from build123d import *

# Parameters (mm, degrees)
F0_R     = 43
F0_R_2   = 40
F0_R_3   = 4.25
F1_DEPTH = 2
F2_DEPTH = 160
F4_DEPTH = 155


with BuildPart() as f1:
    # F0 (on Top) → F1 (new body)
    with BuildSketch(Plane.XY):
        Circle(F0_R)
        Circle(F0_R_2, mode=Mode.SUBTRACT)
        Circle(F0_R_2)
        Circle(F0_R_3, mode=Mode.SUBTRACT)
    extrude(amount=F1_DEPTH)

    # F0 (on Top) → F2 (join)
    with BuildSketch(Plane.XY):
        Circle(F0_R)
        Circle(F0_R_2, mode=Mode.SUBTRACT)
    extrude(amount=F2_DEPTH)

    # F3 (on face) → F4 (cut)
    with BuildSketch(Plane.XY.offset(160)):
        with BuildLine():
            ThreePointArc((-17.935173408, 35.7537348374), (-15.3073372946, 36.9551813005), (-12.5996256178, 37.9637910948))
            Line((-12.5996256178, 37.9637910948), (-15.1896329803, 38.9425798282))
            Line((-15.1896329803, 38.9425798282), (-16.7958697893, 38.2772547575))
            Line((-16.7958697893, 38.2772547575), (-17.935173408, 35.7537348374))
        make_face()
        with BuildLine():
            ThreePointArc((-10.6153464373, 38.5657156036), (-7.8036128806, 39.2314112161), (-4.9511591149, 39.6923925132))
            Line((-4.9511591149, 39.6923925132), (-7.300448003, 41.1576594658))
            Line((-7.300448003, 41.1576594658), (-9.0056199043, 40.8184796861))
            Line((-9.0056199043, 40.8184796861), (-10.6153464373, 38.5657156036))
        make_face()
        with BuildLine():
            Line((-0.8692890969, 41.7910733317), (-2.8875776562, 39.895637547))
            ThreePointArc((-2.8875776562, 39.895637547), (0, 40), (2.8875776562, 39.895637547))
            Line((2.8875776562, 39.895637547), (0.8692890969, 41.7910733317))
            Line((0.8692890969, 41.7910733317), (-0.8692890969, 41.7910733317))
        make_face()
        with BuildLine():
            Line((7.300448003, 41.1576594658), (4.9511591149, 39.6923925132))
            ThreePointArc((4.9511591149, 39.6923925132), (7.8036128806, 39.2314112161), (10.6153464373, 38.5657156036))
            Line((10.6153464373, 38.5657156036), (9.0056199043, 40.8184796861))
            Line((9.0056199043, 40.8184796861), (7.300448003, 41.1576594658))
        make_face()
        with BuildLine():
            Line((15.1896329803, 38.9425798282), (12.5996256178, 37.9637910948))
            ThreePointArc((12.5996256178, 37.9637910948), (15.3073372946, 36.9551813005), (17.935173408, 35.7537348374))
            Line((17.935173408, 35.7537348374), (16.7958697893, 38.2772547575))
            Line((16.7958697893, 38.2772547575), (15.1896329803, 38.9425798282))
        make_face()
        with BuildLine():
            ThreePointArc((-24.5657617227, 31.5677580924), (-22.2228093208, 33.2587844921), (-19.7638955741, 34.7762624751))
            Line((-19.7638955741, 34.7762624751), (-22.4950888807, 35.2309586869))
            Line((-22.4950888807, 35.2309586869), (-23.9406638174, 34.2650563947))
            Line((-23.9406638174, 34.2650563947), (-24.5657617227, 31.5677580924))
        make_face()
        with BuildLine():
            ThreePointArc((-30.2523015911, 26.1686501073), (-28.2842712475, 28.2842712475), (-26.1686501073, 30.2523015911))
            Line((-26.1686501073, 30.2523015911), (-28.9360711307, 30.1654315611))
            Line((-28.9360711307, 30.1654315611), (-30.1654315611, 28.9360711307))
            Line((-30.1654315611, 28.9360711307), (-30.2523015911, 26.1686501073))
        make_face()
        with BuildLine():
            ThreePointArc((-34.7762624751, 19.7638955741), (-33.2587844921, 22.2228093208), (-31.5677580924, 24.5657617227))
            Line((-31.5677580924, 24.5657617227), (-34.2650563947, 23.9406638174))
            Line((-34.2650563947, 23.9406638174), (-35.2309586869, 22.4950888807))
            Line((-35.2309586869, 22.4950888807), (-34.7762624751, 19.7638955741))
        make_face()
        with BuildLine():
            ThreePointArc((-37.9637910948, 12.5996256178), (-36.9551813005, 15.3073372946), (-35.7537348374, 17.935173408))
            Line((-35.7537348374, 17.935173408), (-38.2772547575, 16.7958697893))
            Line((-38.2772547575, 16.7958697893), (-38.9425798282, 15.1896329803))
            Line((-38.9425798282, 15.1896329803), (-37.9637910948, 12.5996256178))
        make_face()
        with BuildLine():
            ThreePointArc((-39.6923925132, 4.9511591149), (-39.2314112161, 7.8036128806), (-38.5657156036, 10.6153464373))
            Line((-38.5657156036, 10.6153464373), (-40.8184796861, 9.0056199043))
            Line((-40.8184796861, 9.0056199043), (-41.1576594658, 7.300448003))
            Line((-41.1576594658, 7.300448003), (-39.6923925132, 4.9511591149))
        make_face()
        with BuildLine():
            Line((22.4950888807, 35.2309586869), (19.7638955741, 34.7762624751))
            ThreePointArc((19.7638955741, 34.7762624751), (22.2228093208, 33.2587844921), (24.5657617227, 31.5677580924))
            Line((24.5657617227, 31.5677580924), (23.9406638174, 34.2650563947))
            Line((23.9406638174, 34.2650563947), (22.4950888807, 35.2309586869))
        make_face()
        with BuildLine():
            Line((28.9360711307, 30.1654315611), (26.1686501073, 30.2523015911))
            ThreePointArc((26.1686501073, 30.2523015911), (28.2842712475, 28.2842712475), (30.2523015911, 26.1686501073))
            Line((30.2523015911, 26.1686501073), (30.1654315611, 28.9360711307))
            Line((30.1654315611, 28.9360711307), (28.9360711307, 30.1654315611))
        make_face()
        with BuildLine():
            Line((34.2650563947, 23.9406638174), (31.5677580924, 24.5657617227))
            ThreePointArc((31.5677580924, 24.5657617227), (33.2587844921, 22.2228093208), (34.7762624751, 19.7638955741))
            Line((34.7762624751, 19.7638955741), (35.2309586869, 22.4950888807))
            Line((35.2309586869, 22.4950888807), (34.2650563947, 23.9406638174))
        make_face()
        with BuildLine():
            Line((38.2772547575, 16.7958697893), (35.7537348374, 17.935173408))
            ThreePointArc((35.7537348374, 17.935173408), (36.9551813005, 15.3073372946), (37.9637910948, 12.5996256178))
            Line((37.9637910948, 12.5996256178), (38.9425798282, 15.1896329803))
            Line((38.9425798282, 15.1896329803), (38.2772547575, 16.7958697893))
        make_face()
        with BuildLine():
            ThreePointArc((-39.895637547, -2.8875776562), (-40, 0), (-39.895637547, 2.8875776562))
            Line((-39.895637547, 2.8875776562), (-41.7910733317, 0.8692890969))
            Line((-41.7910733317, 0.8692890969), (-41.7910733317, -0.8692890969))
            Line((-41.7910733317, -0.8692890969), (-39.895637547, -2.8875776562))
        make_face()
        with BuildLine():
            ThreePointArc((-38.5657156036, -10.6153464373), (-39.2314112161, -7.8036128806), (-39.6923925132, -4.9511591149))
            Line((-39.6923925132, -4.9511591149), (-41.1576594658, -7.300448003))
            Line((-41.1576594658, -7.300448003), (-40.8184796861, -9.0056199043))
            Line((-40.8184796861, -9.0056199043), (-38.5657156036, -10.6153464373))
        make_face()
        with BuildLine():
            ThreePointArc((-35.7537348374, -17.935173408), (-36.9551813005, -15.3073372946), (-37.9637910948, -12.5996256178))
            Line((-37.9637910948, -12.5996256178), (-38.9425798282, -15.1896329803))
            Line((-38.9425798282, -15.1896329803), (-38.2772547575, -16.7958697893))
            Line((-38.2772547575, -16.7958697893), (-35.7537348374, -17.935173408))
        make_face()
        with BuildLine():
            ThreePointArc((-31.5677580924, -24.5657617227), (-33.2587844921, -22.2228093208), (-34.7762624751, -19.7638955741))
            Line((-34.7762624751, -19.7638955741), (-35.2309586869, -22.4950888807))
            Line((-35.2309586869, -22.4950888807), (-34.2650563947, -23.9406638174))
            Line((-34.2650563947, -23.9406638174), (-31.5677580924, -24.5657617227))
        make_face()
        with BuildLine():
            ThreePointArc((-26.1686501073, -30.2523015911), (-28.2842712475, -28.2842712475), (-30.2523015911, -26.1686501073))
            Line((-30.2523015911, -26.1686501073), (-30.1654315611, -28.9360711307))
            Line((-30.1654315611, -28.9360711307), (-28.9360711307, -30.1654315611))
            Line((-28.9360711307, -30.1654315611), (-26.1686501073, -30.2523015911))
        make_face()
        with BuildLine():
            ThreePointArc((-19.7638955741, -34.7762624751), (-22.2228093208, -33.2587844921), (-24.5657617227, -31.5677580924))
            Line((-24.5657617227, -31.5677580924), (-23.9406638174, -34.2650563947))
            Line((-23.9406638174, -34.2650563947), (-22.4950888807, -35.2309586869))
            Line((-22.4950888807, -35.2309586869), (-19.7638955741, -34.7762624751))
        make_face()
        with BuildLine():
            ThreePointArc((-12.5996256178, -37.9637910948), (-15.3073372946, -36.9551813005), (-17.935173408, -35.7537348374))
            Line((-17.935173408, -35.7537348374), (-16.7958697893, -38.2772547575))
            Line((-16.7958697893, -38.2772547575), (-15.1896329803, -38.9425798282))
            Line((-15.1896329803, -38.9425798282), (-12.5996256178, -37.9637910948))
        make_face()
        with BuildLine():
            ThreePointArc((-4.9511591149, -39.6923925132), (-7.8036128806, -39.2314112161), (-10.6153464373, -38.5657156036))
            Line((-10.6153464373, -38.5657156036), (-9.0056199043, -40.8184796861))
            Line((-9.0056199043, -40.8184796861), (-7.300448003, -41.1576594658))
            Line((-7.300448003, -41.1576594658), (-4.9511591149, -39.6923925132))
        make_face()
        with BuildLine():
            ThreePointArc((2.8875776562, -39.895637547), (0, -40), (-2.8875776562, -39.895637547))
            Line((-2.8875776562, -39.895637547), (-0.8692890969, -41.7910733317))
            Line((-0.8692890969, -41.7910733317), (0.8692890969, -41.7910733317))
            Line((0.8692890969, -41.7910733317), (2.8875776562, -39.895637547))
        make_face()
        with BuildLine():
            Line((9.0056199043, -40.8184796861), (10.6153464373, -38.5657156036))
            ThreePointArc((10.6153464373, -38.5657156036), (7.8036128806, -39.2314112161), (4.9511591149, -39.6923925132))
            Line((4.9511591149, -39.6923925132), (7.300448003, -41.1576594658))
            Line((7.300448003, -41.1576594658), (9.0056199043, -40.8184796861))
        make_face()
        with BuildLine():
            Line((16.7958697893, -38.2772547575), (17.935173408, -35.7537348374))
            ThreePointArc((17.935173408, -35.7537348374), (15.3073372946, -36.9551813005), (12.5996256178, -37.9637910948))
            Line((12.5996256178, -37.9637910948), (15.1896329803, -38.9425798282))
            Line((15.1896329803, -38.9425798282), (16.7958697893, -38.2772547575))
        make_face()
        with BuildLine():
            Line((40.8184796861, 9.0056199043), (38.5657156036, 10.6153464373))
            ThreePointArc((38.5657156036, 10.6153464373), (39.2314112161, 7.8036128806), (39.6923925132, 4.9511591149))
            Line((39.6923925132, 4.9511591149), (41.1576594658, 7.300448003))
            Line((41.1576594658, 7.300448003), (40.8184796861, 9.0056199043))
        make_face()
        with BuildLine():
            Line((41.7910733317, 0.8692890969), (39.895637547, 2.8875776562))
            ThreePointArc((39.895637547, 2.8875776562), (39.9739008722, 1.4447314839), (40, 0))
            ThreePointArc((40, 0), (39.9739008722, -1.4447314839), (39.895637547, -2.8875776562))
            Line((39.895637547, -2.8875776562), (41.7910733317, -0.8692890969))
            Line((41.7910733317, -0.8692890969), (41.7910733317, 0.8692890969))
        make_face()
        with BuildLine():
            Line((41.1576594658, -7.300448003), (39.6923925132, -4.9511591149))
            ThreePointArc((39.6923925132, -4.9511591149), (39.2314112161, -7.8036128806), (38.5657156036, -10.6153464373))
            Line((38.5657156036, -10.6153464373), (40.8184796861, -9.0056199043))
            Line((40.8184796861, -9.0056199043), (41.1576594658, -7.300448003))
        make_face()
        with BuildLine():
            Line((38.9425798282, -15.1896329803), (37.9637910948, -12.5996256178))
            ThreePointArc((37.9637910948, -12.5996256178), (36.9551813005, -15.3073372946), (35.7537348374, -17.935173408))
            Line((35.7537348374, -17.935173408), (38.2772547575, -16.7958697893))
            Line((38.2772547575, -16.7958697893), (38.9425798282, -15.1896329803))
        make_face()
        with BuildLine():
            Line((35.2309586869, -22.4950888807), (34.7762624751, -19.7638955741))
            ThreePointArc((34.7762624751, -19.7638955741), (33.2587844921, -22.2228093208), (31.5677580924, -24.5657617227))
            Line((31.5677580924, -24.5657617227), (34.2650563947, -23.9406638174))
            Line((34.2650563947, -23.9406638174), (35.2309586869, -22.4950888807))
        make_face()
        with BuildLine():
            Line((30.1654315611, -28.9360711307), (30.2523015911, -26.1686501073))
            ThreePointArc((30.2523015911, -26.1686501073), (28.2842712475, -28.2842712475), (26.1686501073, -30.2523015911))
            Line((26.1686501073, -30.2523015911), (28.9360711307, -30.1654315611))
            Line((28.9360711307, -30.1654315611), (30.1654315611, -28.9360711307))
        make_face()
        with BuildLine():
            Line((23.9406638174, -34.2650563947), (24.5657617227, -31.5677580924))
            ThreePointArc((24.5657617227, -31.5677580924), (22.2228093208, -33.2587844921), (19.7638955741, -34.7762624751))
            Line((19.7638955741, -34.7762624751), (22.4950888807, -35.2309586869))
            Line((22.4950888807, -35.2309586869), (23.9406638174, -34.2650563947))
        make_face()
    extrude(amount=-F4_DEPTH, mode=Mode.SUBTRACT)


solid = f1.part
Geometry: final body of the model. Coordinates: model frame, mm. Give positions to 0.01 mm unless a question says otherwise; leave off trailing zeros. Put each result on its own line as item: value.
1) First-contact query: P1, Ø1.1, axis at x = 33.5, y = 22.5, coming from the +Z side; P2, Ø5, axis at x = -34, z = 60.5, coming from the -Y side; P3, Ø13.5, axis at x = 0, y = 0, coming from the +Z side. Flat tips, straight axial feed; report the tip coordinate or a pass-through.
Computed values:
P1: stops at z = 5
P2: stops at y = -29.27
P3: stops at z = 2
2) Material intervals for L1, parallel to Y at x = 0, z = 94; L2, parallel to Y at x = 0, z = 0.95; L3, parallel to X at y = -29, z = 129, sorted ascending. Write a range as from..to.
Computed values:
L1: y = -43..-41.79, 41.79..43
L2: y = -43..-4.25, 4.25..43
L3: x = -31.75..-30.1, 30.1..31.75
3) Mould query, pull axis Y, two halves, no side actions, for faces 1 (the flat face through (38, -15, 5)), 2 (the flat face through (-35.24, 19.31, 160)), 3 (the cylindrical face through (-5.598, 42.634, 78.88)). Classes: released by +Y, released by -Y, zero draft, split by the parting line, or undercut.
Computed values:
face 1: undercut
face 2: zero draft
face 3: split by the parting line
